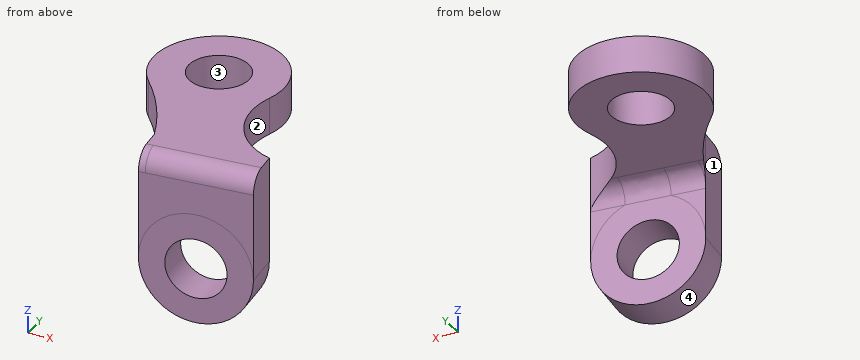
Autodesk Inventor part; units mm, degrees
ref_plane "LinkPlane" through (14.2753, -15.8345, 0) normal (-0.124003, 0.9922818, 0) x (0.9625852, 0.1202919, 0.2428158)
ref_plane "LowerMountPlane" through (0, 0, 0) normal (0, 0, -1) x (-1, 0, 0)
ref_plane "YZ Plane" through (0, 0, 0) normal (1, 0, 0) x (0, 1, 0)
sketch "Base" plane through (0, 0, 0) normal (0, 0, 1) x (1, 0, 0)
  circle A0 centre (0, 0) radius 3.25
  circle A1 centre (0, 0) radius 7
  dimension "d0" = 6.5
  dimension "d1" = 14
extrude "BaseFeature" add sketch "Base" along normal blind 4
ref_plane "LinkPlane" through (14.2753, -15.8345, 0) normal (-0.124003, 0.9922818, 0) x (0.9625852, 0.1202919, 0.2428158)
sketch "LinkEnd" plane through (14.2753, -15.8345, 0) normal (-0.124003, 0.9922818, 0) x (0.9625852, 0.1202919, 0.2428158)
  line L0 (-6.4275, 8.6997) -> (-5.2135, 3.8493) construction
  line L1 (-8.3662, 3.0601) -> (-9.5803, 7.9105) construction
  line L2 (-8.3662, 3.0601) -> (-5.2135, 3.8493) construction
  circle A0 centre (-8.9732, 5.4853) radius 3.25
  circle A1 centre (-8.9732, 5.4853) radius 6
  dimension "d21" = 5
  dimension "d23" = 3.25
  dimension "d24" = 5
  dimension "d25" = 6.5
  dimension "d26" = 12
extrude "LinkEndFeature" add sketch "LinkEnd" along normal blind 4
ref_plane "LowerMountPlane" through (0, 0, 0) normal (0, 0, -1) x (-1, 0, 0)
sketch "LowerMount" plane through (0, 0, 0) normal (0, 0, -1) x (-1, 0, 0)
  line L0 (-9.6884, -12.3766) -> (-3.2385, -13.1827)
  line L1 (-0.5098, -13.5237) -> (-12.4171, -12.0356)
  circle A0 centre (0, 0) radius 7
  arc A1 (5.0617, -4.8352) -> (-0.5098, -13.5237) centre (24.5854, -23.4853) ccw
  arc A2 (-12.4171, -12.0356) -> (-6.7091, -1.997) centre (-14.3766, -4.2793) ccw
  arc A3 (-6.7091, -1.997) -> (5.0617, -4.8352) centre (0, 0) ccw
  dimension "d27" = 8
  dimension "d28" = 27
extrude "LowerMountFeature" add sketch "LowerMount" against normal up to surface (4 mm away) contours L1 A2 A0 A1 L0
sketch "Link" plane through (6.9595, -16.7488, -7.5) normal (0.124003, -0.9922818, 0) x (0.9922818, 0.124003, 0)
  line L0 (6, 11.5) -> (-6, 11.5)
  line L1 (-6, 7.5) -> (-6, 11.5)
  line L2 (6, 7.5) -> (-6, 7.5)
  line L3 (6, 7.5) -> (6, 11.5)
  circle A0 centre (0, 0) radius 6
  line L4 (6, 7.5) -> (6, 0)
  line L5 (-6, 0) -> (-6, 7.5)
extrude "LinkFeature" add sketch "Link" against normal up to surface (4 mm away) contours L3 L2 L1 L0 | L4 A0 L5 L2
fillet "LinkFilletsFeature" radius 2 2 edges at (6.4635, -12.7797, 0) (6.9595, -16.7488, 4)
properties part number "ElbowConnectorUnderlinkLeft"
The listing builds one solid part. Answer for the finished solid, in the listing's coordinates (mm). Face numbers are marked on the shaded views. Coordinates: 2 decimals unless noted, no trailing zeros. Write each loop counter-clockwise with the first axis right and the second up, starting at its lowest first coordinate (ties: lowest second). Pieces come first, ordered by that corner, then holes. Notation, with made-up numbers: (49, 69) - (70, 69) arc R19 ccw to (70, 84) - close; hole circle Ø11 at (30.25, 15). An arc over 180 degrees is marked (long way). Answer as CSV lines item,"result".
1. Given P1, Ø6, axis at x = -4.5, z = -1.5, coming from the -Y side; P2, Ø1, axis at x = 8, y = -6, coming from the -Z side; P3, Ø8, axis at x = 1.5, y = -3, coming from the -Z side; P4, Ø10, axis at y = -9, z = -1, coming from the -X side, each flat-ended and moving along its own axis, determine where each tip first touches the part or whether it passes through.
Computed values:
P1,"stops at y = -8.84"
P2,"passes through"
P3,"stops at z = 0"
P4,"stops at x = -5.67"
2. Determine the mould class of the marked faces 1, 2, 3 and 4 for opening direction Y: +Y half, -Y half, draft (parallel to the pull), parting line (faces both ways), or undercut.
Computed values:
face 1,"-Y half"
face 2,"undercut"
face 3,"undercut"
face 4,"parting line"
3. Straight lines are drawn through the part: line 1 (X direction, y = 0, z = 1.05); line 2 (Z direction, x = 2.5, y = -5); line 3 (Z direction, x = 4.75, y = -13.5). For each, find the intervals that lie inside material, in ascending order. Write a range as [from, to].
Computed values:
line 1,"x = [-7, -3.25], [3.25, 7]"
line 2,"z = [0, 4]"
line 3,"z = [-13.23, -10.21], [-4.79, 4]"
4. Find section D-D (y = -8.75). Give the vertices of the cut face in (x, z), plus the area to 3 significant figures.
Computed values:
outline,"(-1.96, 0) - (7.74, 0) - (7.74, 4) - (-1.96, 4) - close"
area,"38.8 mm²"
5. Find section B-B (y = 0). Give the vertices of the cut face in (x, z).
Computed values:
outline,"(-7, 0) - (-3.25, 0) - (-3.25, 4) - (-7, 4) - close; (3.25, 0) - (7, 0) - (7, 4) - (3.25, 4) - close"
6. Find section A-A (x = -1.5). Give the vertices of the cut face in (y, z).
Computed values:
outline,"(-9.48, 0) - (-2.88, 0) - (-2.88, 4) - (-9.48, 4) - close; (2.88, 0) - (6.84, 0) - (6.84, 4) - (2.88, 4) - close"
7. Find section C-C (z = -5). Give the vertices of the cut face in (x, y).
Computed values:
outline,"(0.51, -13.52) - (1.01, -17.49) - (4.9, -17.01) - (4.4, -13.04) - close; (8.52, -12.52) - (9.02, -16.49) - (12.91, -16) - (12.42, -12.04) - close"
